Read the model definition and answer for the solid it produces. Units are mm, in the model's axes. A direction names the side the tool comes from. Give positions to 0.01 mm unless a question says otherwise; leave off trailing zeros. Order: outer loops, then holes, each group sorted by start corner. A loop starts at its lowest first (then second) coordinate and runs counter-clockwise, first axis right, second up. Notation, with made-up numbers: (-34, 3.25) -> (-4, 3.25) arc R31 ccw to (-4, 35.25) -> close; hole circle Ø1 at (-6.75, 12.5). An arc over 180 degrees is marked (long way). One line per item, written item: value. Start each with the question number.
Autodesk Inventor part; units mm, degrees
ref_plane "Work Plane1" through (20.959, 0, 0) normal (0, 0, -1) x (-1, 0, 0)
ref_plane "YZ Plane" through (0, 0, 0) normal (1, 0, 0) x (0, 1, 0)
ref_plane "XZ Plane" through (0, 0, 0) normal (0, 1, 0) x (-1, 0, 0)
sketch "Sketch1" plane through (0, 0, 0) normal (0, 0, 1) x (1, 0, 0)
  line L0 (-1.4239, 0) -> (7.2373, 0)
  line L1 (2.78, 5) -> (2.0969, 6.4649)
  line L2 (2.78, 5) -> (6, 5) construction
  line L3 (6, 5) -> (6, 0) construction
  arc A0 (2.0969, 6.4649) -> (0, 6) centre (1.1, 6) ccw
  line L4 (2.78, 5) -> (2.78, 0)
  line L5 (0, -1.4613) -> (0, 8.7676)
  point P0 (0, 0)
  dimension "d2" = 10
  dimension "d4" = 14.2
  dimension "d5" = 1.1
  dimension "d15" = 6
  dimension "d16" = 25
revolve "Ring" add sketch "Sketch1" angle 360 about axis through (-10, 0, 0) along (1, 0, 0)
sketch "Sketch2" plane through (0, 0, 0) normal (-1, 0, 0) x (0, 0, 1)
  circle A0 centre (0, 0) radius 4.9
  line L0 (-5, -2.8868) -> (-5, 2.8868)
  line L1 (-5, 2.8868) -> (0, 5.7735)
  line L2 (0, 5.7735) -> (5, 2.8868)
  line L3 (5, 2.8868) -> (5, -2.8868)
  line L4 (5, -2.8868) -> (0, -5.7735)
  line L5 (0, -5.7735) -> (-5, -2.8868)
  circle A1 centre (0, 0) radius 6
  dimension "d6" = 11.547
extrude "Body" add sketch "Sketch2" against normal blind 6 contours A0 | L0 L1 L2 L3 L4 L5
sketch "Sketch3" plane through (0, 0, 0) normal (0, 0, 1) x (1, 0, 0)
  line L0 (2.4193, 5.7735) -> (6, 5.7735)
  line L1 (6, 2.8868) -> (6, 5.7735)
  line L2 (0, -6) -> (0, 6)
  line L3 (-1.2, 0) -> (7.2, 0)
  line L4 (5.7927, 5.7735) -> (6, 5)
  dimension "d10" = 15
  dimension "d11" = 10
revolve "Chamfer1" cut sketch "Sketch3" angle 360 about axis through (-10, 0, 0) along (1, 0, 0)
sketch "Sketch4" plane through (0, 0, 0) normal (-1, 0, 0) x (0, 0, 1)
  circle A0 centre (0, 0) radius 6
hole "Thread" at (0, 0, 0) direction (1, 0, 0) diameter 4.917 end through all
chamfer "Chamfer2" distance 0.5413 angle 30 1 edges at (0, 0, -2.4585) measured on face at (0, 4.7554, -0.5774)
ref_plane "Work Plane1" through (20.959, 0, 0) normal (0, 0, -1) x (-1, 0, 0)
chamfer "Chamfer3" distance 0.5413 angle 45 1 edges at (6, 0, -2.4585)
equation "\"d2\" = SW"
equation "\"d4\" = LADI"
equation "\"d5\" = PHH"
equation "\"d15\" = KOH"
equation "\"d16\" = KEWI"
equation "\"d6\" = 1.1547 * SW"
equation "\"d7\" = KOH"
equation "\"d10\" = ANG1"
equation "\"d11\" = SW0"
equation "\"d12\" = -0.5 * GD1 + 0.5 * NND"
equation "\"d46\" = -0.5 * GD1 + 0.5 * NND"
equation "\"d51\" = -0.5 * GD1 + 0.5 * NND"
equation "\"ANG1\" = 15deg"
equation "\"KEWI\" = 25deg"
equation "\"NND\" = 6"
equation "\"LADI\" = 14.2"
equation "\"SW\" = 10"
equation "\"PHH\" = RR"
equation "\"KOH\" = NND"
equation "\"SW0\" = SW"
equation "\"d1\" = LADI"
equation "\"d3\" = PHH"
equation "\"GUL\" = 0.541266 * PTC"
equation "\"RR\" = 1.1"
equation "\"THREADDIA\" = 6"
equation "\"TOA\" = 30deg"
equation "\"PTC\" = 1"
equation "\"GAL\" = 0.541266 * PTC"
equation "\"E0\" = 1.155 * SW"
properties part number "DIN 6923 - M6" material "Steel, Mild"
Item 1: For a pull along Y with two mould halves and no side action, classify faces 4 (the flat face through (4.185, -4.31, 2.535)), 5 (the flat face through (0, -3, -1)), 6 (the cylindrical face through (2.922, -0.738, 2.345)), 7 (the conical face through (5.95, 5.19, 0.01)) as +Y half, -Y half, draft (parallel to the pull), parting line (faces both ways), or undercut.
Item 2: Find the intervals of material crossed by line 1 (Z direction, x = 3.2, y = 0); line 2 (Y direction, x = 3.5, z = 1.5); line 3 (Y direction, x = 0.5, z = -1.5), in increasing order. Write a range as from..to.
Item 3: Find section A-A on x = 3. Write down the section's boundary in (y, z).
Item 4: Flat-ended cylindrical pins translate along their axes: pin 1 (1 mm diameter, centred on x = 3.5, y = 2, fed in from +Z); pin 2 (3 mm diameter, centred on x = 1.5, y = -4, fed in from +Z). Find the tip coordinate at first contact, or state that the pin passes through.
Item 5: A tool of negligible diameter and unlimited length cuts with its end or side. For faces 1 (the flat face through (4.185, 4.35, 2.465)), 2 (the flat face through (4.185, 4.31, -2.535)), 3 (the flat face through (4.185, -4.35, -2.465)), from which of +Z, -Z, +X, -X, +Y, -Y can it reach the whole face along a straight path? Write none if from no direction.
Item 6: Find section B-B on x = 1.25. Write down the section's boundary in (y, z), then the cut area to 3 significant figures.
Checks:
1. face 4: -Y half
1. face 5: draft
1. face 6: undercut
1. face 7: +Y half
2. line 1: -5..-2.46, 2.46..5
2. line 2: -4.91..-1.95, 1.95..4.91
2. line 3: -6.76..-1.95, 1.95..6.76
3. outline: (-5.77, 0) -> (-2.89, -5) -> (2.89, -5) -> (5.77, 0) -> (2.89, 5) -> (-2.89, 5) -> close; hole circle Ø4.92 at (0, 0)
4. pin 1: z = 5
4. pin 2: z = 6.63
5. face 1: +Z, +X, +Y
5. face 2: -Z, +X, +Y
5. face 3: -Z, +X, -Y
6. outline: circle Ø14.18 at (0, 0); hole circle Ø4.92 at (0, 0)
6. area: 139 mm2
